Could you check a few things on this drawing? It's one solid part, dimensions in mm from its lowest x, y, z. Coordinates: 2 decimals unless noted, no trailing zeros. Order: outer loops, then holes, each group sorted by start corner. A loop starts at its lowest first (then second) coordinate and runs counter-clockwise, first axis right, second up.
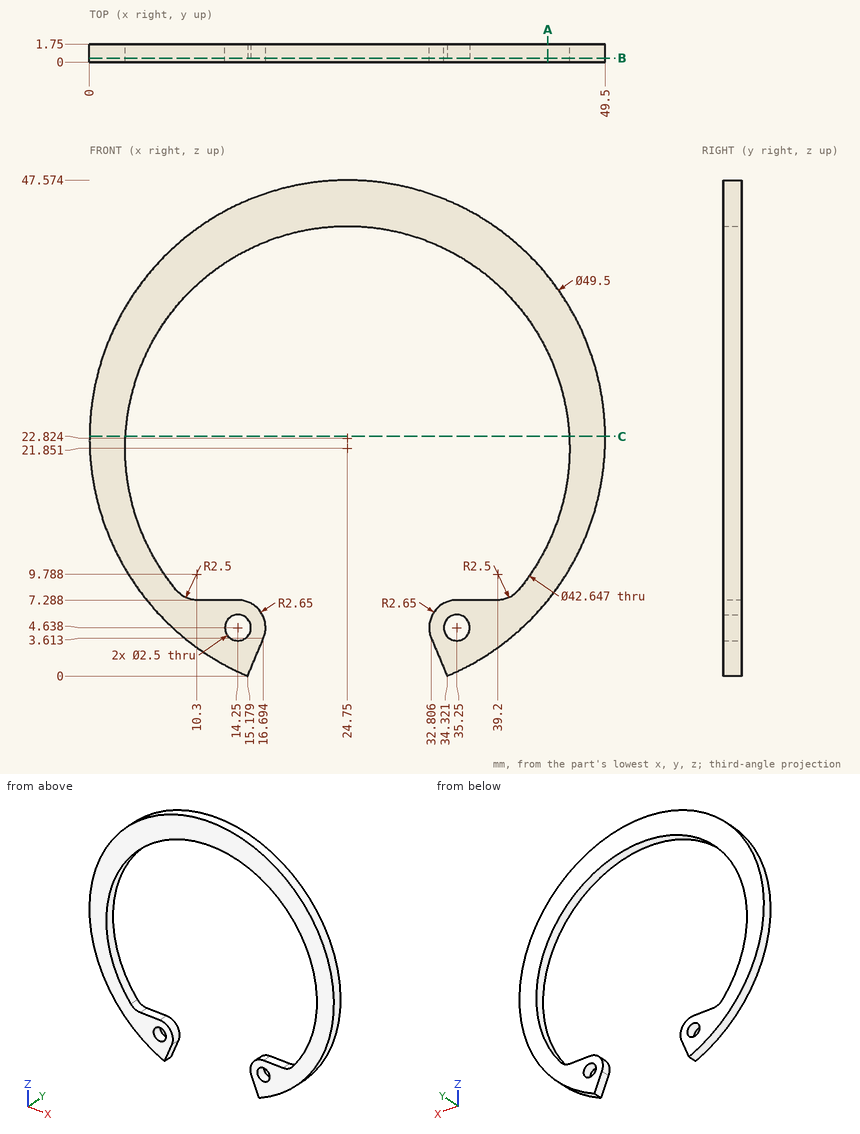
1. Imagine slicing it at C-C on z = 23. Please give me the cut outline in (x, y).
Completed:
outline: (0, 0) - (3.46, 0) - (3.46, 1.75) - (0, 1.75) - close; (46.04, 0) - (49.5, 0) - (49.5, 1.75) - (46.04, 1.75) - close
2. I'm going to push flat-ended pins straight in: pin 1 (0.9 mm diameter, centred on x = 37, y = 0.5, fed in from +Z); pin 2 (1.5 mm diameter, centred on x = 14.25, z = 4.64, fed in from -Y). Where does each tip first touch, or does it pass through?
Completed:
pin 1: stops at z = 44.58
pin 2: passes through
3. Imagine slicing it at A-A on x = 44. Please give me the cut outline in (y, z).
Completed:
outline: (0, 7.27) - (1.75, 7.27) - (1.75, 12.68) - (0, 12.68) - close; (0, 31.02) - (1.75, 31.02) - (1.75, 38.38) - (0, 38.38) - close
4. Imagine slicing it at B-B on y = 0.4. Give the number of separate pieces and of enclosed holes in the cut face, then the cut area to 3 significant figures.
Completed:
separate pieces: 1
enclosed holes: 2
area: 483 mm2
5. Please list where these lines run through material, in increasing order: probe 1 along Z at (x, y) = (44, 0.35) (1 decimal); probe 2 along X at (y, z) = (0.75, 28.5); probe 3 along X at (y, z) = (0.5, 2.5) (1 decimal).
Completed:
probe 1: z = 7.3 to 12.7, 31 to 38.4
probe 2: x = 0.66 to 4.49, 45.01 to 48.84
probe 3: x = 10.6 to 16.2, 33.3 to 38.9
